The listing builds one solid part. Answer for the finished solid, in the listing's coordinates (mm). A direction names the side the tool comes from. Coordinates: 2 decimals unless noted, no trailing zeros. Order: outer loops, then holes, each group sorted by start corner. A loop starts at its lowest first (then second) coordinate and runs counter-clockwise, first axis right, second up. Notation, with made-up numbers: (-15, 52.5) - (23, 52.5) arc R35 ccw to (23, 88.5) - close; hole circle Ø7 at (87, -38). An arc over 180 degrees is marked (long way). Use one line per item in the form item = value. Start each with the question number.
Item 1: A tool of negligible diameter and unlimited length cuts with its end or side. For faces 1 (the flat face through (-15, 0, 24)), 2 (the flat face through (-1, 10, 0)), from which of +Z, -Z, +X, -X, +Y, -Y can it reach the whole face along a straight path? Write none if from no direction.
Item 2: Section B-B, the plane z = 0 is taken. Write down the section's boundary in (x, y).
Item 3: Each of these flat-tipped pins is pushed along its axis until it touches: pin 1 Ø2.5 at (x, z) = (38.4, 0) entering from +Y; pin 2 Ø1 at (x, z) = (33.5, -1.5) entering from -Y. Where does it stop, or does it pass through?
Item 4: The mould has two halves that part along Z. Classify faces 3 (the flat face through (-1, 6, 25.45)), 4 (the flat face through (-1, 12, 0)), 5 (the flat face through (-1, 6, -25.45)), 6 (the flat face through (-48.9, 4, 0)): released by +Z, released by -Z, zero draft, split by the parting line, or undercut.
Item 5: Section A-A, the plane x = 38.4 is taken. Write down the section's boundary in (y, z), and give its area (3 significant figures).
Item 6: Section D-D, the plane z = 11 is taken. Write down the section's boundary in (x, y), and give its area (3 significant figures).
Item 7: Section C-C, the plane y = 6.5 is taken. Write down the section's boundary in (x, z).
Item 8: Consider line 1 along X through (y, z) = (11.2, 0); line 2 along X through (y, z) = (4.25, -0.5); line 3 along Z through (x, y) = (7.5, 2.5). Determine where each line is inside the solid, lowest interval first. Write a range as [from, to].
from build123d import *

# Parameters (mm, degrees)
SKETCH1_W             = 101.8
SKETCH1_H             = 50.9
SKETCH1_W_2           = 97.8
SKETCH1_H_2           = 46.9
MAIN_BODY_DEPTH       = 10
SKETCH4_W             = 101.8
SKETCH4_H             = 50.9
TOP_DEPTH             = 2
OUTER_FILLET_0_2MM_R  = 0.4
INNER_FILLET_1MM_R    = 1
HOLES_CUT_4_2MM_REACH = 60.159
SKETCH6_R             = 2.1


with BuildPart() as part:
    # Sketch1 → Main Body (new body)
    with BuildSketch(Plane(origin=(0, 0, 0), x_dir=(1, 0, 0), z_dir=(0, 1, 0))):
        Rectangle(SKETCH1_W, SKETCH1_H)
        Rectangle(SKETCH1_W_2, SKETCH1_H_2, mode=Mode.SUBTRACT)
    extrude(amount=MAIN_BODY_DEPTH)

    # Sketch4 → Top (add)
    with BuildSketch(Plane(origin=(0, 10, 0), x_dir=(1, 0, 0), z_dir=(0, 1, 0))):
        Rectangle(SKETCH4_W, SKETCH4_H)
    extrude(amount=TOP_DEPTH)

    # Outer Fillet 0.2mm
    outer_fillet_0_2mm_edges = [part.edges().sort_by_distance(p)[0] for p in [
        (0, 12, -25.45),
        (-50.9, 12, 0),
        (0, 12, 25.45),
        (50.9, 12, 0),
        (-50.9, 6, -25.45),
        (50.9, 6, -25.45),
        (50.9, 6, 25.45),
        (-50.9, 6, 25.45),
    ]]
    fillet(outer_fillet_0_2mm_edges, radius=OUTER_FILLET_0_2MM_R)

    # Inner Fillet 1mm
    inner_fillet_1mm_edges = [part.edges().sort_by_distance(p)[0] for p in [
        (48.9, 5, -23.45),
        (-48.9, 5, -23.45),
        (-48.9, 5, 23.45),
        (48.9, 5, 23.45),
        (0, 10, -23.45),
        (-48.9, 10, 0),
        (0, 10, 23.45),
        (48.9, 10, 0),
    ]]
    fillet(inner_fillet_1mm_edges, radius=INNER_FILLET_1MM_R)

    # Sketch6 → Holes Cut 4.2mm (cut, up to next)
    with BuildSketch(Plane(origin=(0, 12, 0), x_dir=(1, 0, 0), z_dir=(0, 1, 0)), mode=Mode.PRIVATE) as holes_cut_4_2mm_sk1:
        with Locations(Location((-38.4, 0, 0), (0, 0, 270))):
            Circle(SKETCH6_R)
    holes_cut_4_2mm_tool1 = extrude(holes_cut_4_2mm_sk1.sketch, amount=-HOLES_CUT_4_2MM_REACH, mode=Mode.PRIVATE) & part.part
    # Sketch6 → Holes Cut 4.2mm (cut, up to next)
    with BuildSketch(Plane(origin=(0, 12, 0), x_dir=(1, 0, 0), z_dir=(0, 1, 0)), mode=Mode.PRIVATE) as holes_cut_4_2mm_sk2:
        with Locations(Location((38.4, 0, 0), (0, 0, 270))):
            Circle(SKETCH6_R)
    holes_cut_4_2mm_tool2 = extrude(holes_cut_4_2mm_sk2.sketch, amount=-HOLES_CUT_4_2MM_REACH, mode=Mode.PRIVATE) & part.part
    add(holes_cut_4_2mm_tool1.solids().sort_by_distance((-38.4, 12, 0))[0], mode=Mode.SUBTRACT)
    add(holes_cut_4_2mm_tool2.solids().sort_by_distance((38.4, 12, 0))[0], mode=Mode.SUBTRACT)


solid = part.part
Response:
q1.face_1 = +Z, -Z, +X, -X, -Y
q1.face_2 = -Y
q2.outline = (-50.9, 0) - (-48.9, 0) - (-48.9, 9) arc R1 cw to (-47.9, 10) - (-40.5, 10) - (-40.5, 12) - (-50.5, 12) arc R0.4 ccw to (-50.9, 11.6) - close; (-36.3, 10) - (36.3, 10) - (36.3, 12) - (-36.3, 12) - close; (40.5, 10) - (47.9, 10) arc R1 cw to (48.9, 9) - (48.9, 0) - (50.9, 0) - (50.9, 11.6) arc R0.4 ccw to (50.5, 12) - (40.5, 12) - close
q3.pin_1 = through
q3.pin_2 = 10
q4.face_3 = released by +Z
q4.face_4 = zero draft
q4.face_5 = released by -Z
q4.face_6 = undercut
q5.outline = (0, -25.45) - (11.6, -25.45) arc R0.4 ccw to (12, -25.05) - (12, -2.1) - (10, -2.1) - (10, -22.45) arc R1 cw to (9, -23.45) - (0, -23.45) - close; (0, 23.45) - (9, 23.45) arc R1 cw to (10, 22.45) - (10, 2.1) - (12, 2.1) - (12, 25.05) arc R0.4 ccw to (11.6, 25.45) - (0, 25.45) - close
q5.area = 134 mm2
q6.outline = (-50.9, 0) - (-48.9, 0) - (-48.9, 9) arc R1 cw to (-47.9, 10) - (47.9, 10) arc R1 cw to (48.9, 9) - (48.9, 0) - (50.9, 0) - (50.9, 11.6) arc R0.4 ccw to (50.5, 12) - (-50.5, 12) arc R0.4 ccw to (-50.9, 11.6) - close
q6.area = 244 mm2
q7.outline = (-50.9, -25.05) arc R0.4 ccw to (-50.5, -25.45) - (50.5, -25.45) arc R0.4 ccw to (50.9, -25.05) - (50.9, 25.05) arc R0.4 ccw to (50.5, 25.45) - (-50.5, 25.45) arc R0.4 ccw to (-50.9, 25.05) - close; hole (-48.9, -22.45) arc R1 ccw to (-47.9, -23.45) - (47.9, -23.45) arc R1 ccw to (48.9, -22.45) - (48.9, 22.45) arc R1 ccw to (47.9, 23.45) - (-47.9, 23.45) arc R1 ccw to (-48.9, 22.45) - close
q8.line_1 = [-50.9, -40.5], [-36.3, 36.3], [40.5, 50.9]
q8.line_2 = [-50.9, -48.9], [48.9, 50.9]
q8.line_3 = [-25.45, -23.45], [23.45, 25.45]
